Design review of the part shown in the three views and the two pictorial views. Dimensions are in mm from the part's minimum x, y and z. A direction names the side the tool comes from. Round coordinates to 2 decimals unless told otherwise and drop trailing zeros. Order: outer loops, then holes, each group sorted by start corner. A loop starts at its lowest first (then second) coordinate and runs counter-clockwise, first axis right, second up. Notation, with made-up numbers: M 76.5,68.5 L 114.5,68.5 A17 cw 114.5,84.5 Z; hole C 84,26.5 d4. An arc over 180 degrees is marked long. Write item = value, one per line. Start each with the question number.
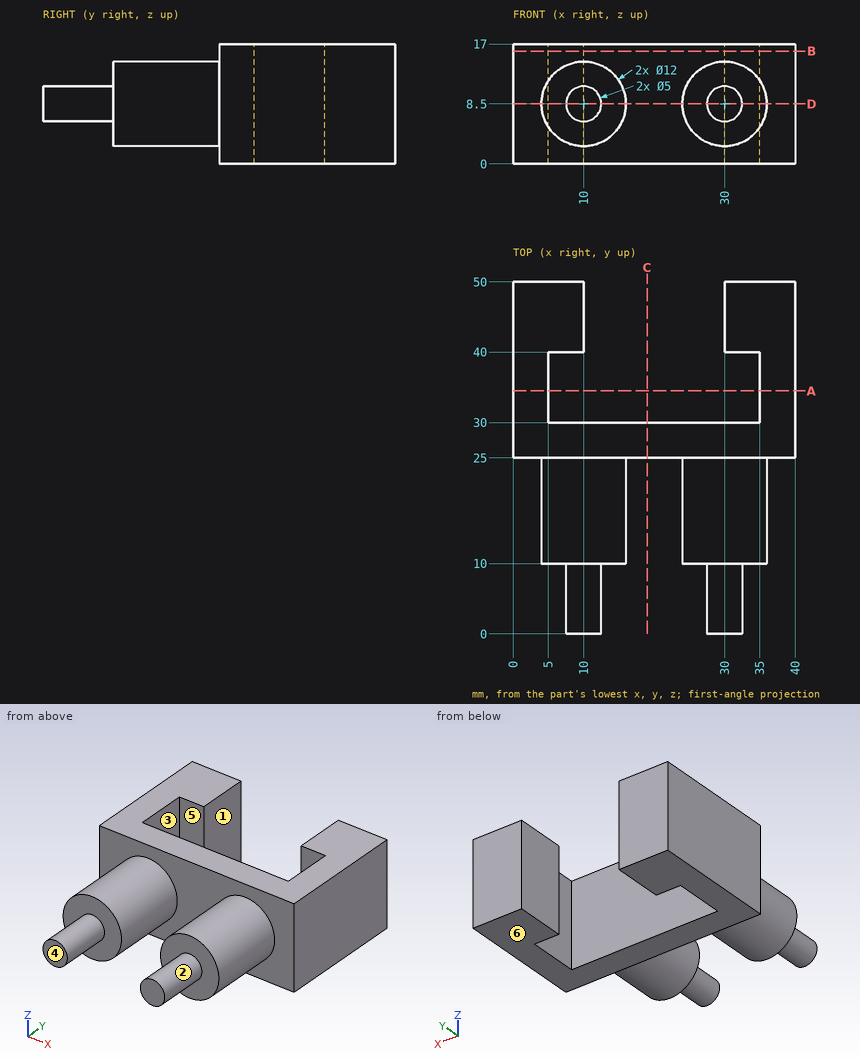
(1) For the marked faces 1, 2 and 3, list the 3-axis set-ups (+Z, -Z, +X, -X, +Y, -Y) from which the entire face can be reached by the end or side of a thin tool; tool diameter is ignored.
(2) For line 1 along X through (y, z) = (6.5, 8.75); line 2 along X through (y, z) = (31, 9.25); line 3 along Y through (x, z) = (11, 11.25), list the stretches that pass through material, from the lowest coordinate up.
(3) We need section A-A, the plane y = 34.5. Write out the cut boundary in (x, z), then the cut area to 3 significant figures.
(4) We need section B-B, the plane z = 16. Write out the cut boundary in (x, y), then the cut area to 3 significant figures.
(5) Draft analysis for pull direction Y (two halves, no side actions). For the marked faces 4, 5 and 6, state which applies: released by +Y, released by -Y, zero draft, split by the parting line, or undercut.
(6) We need section C-C, the plane x = 19. Write out the cut boundary in (y, z).
(7) We need section D-D, the plane z = 8.5. Write out the cut boundary in (x, y), then the cut area to 3 significant figures.
(8) Insertion check: pin 1 (5 mm diameter, centred on y = 47.5, z = 9.5, fed in from -X); pin 2 (2.5 mm diameter, centred on x = 7.5, z = 12.5, fed in from -Y); pin 3 (8.5 mm diameter, centred on x = 16.5, z = 5.5, fed in from +Y); pin 4 (4 mm diameter, centred on y = 22.5, z = 7.5, fed in from -X). Each pin has a flat end and moves straight along its axis. Give the tip position at first contact, or say it passes through.
Values:
q1.face_1 = +Z, -Z, +Y
q1.face_2 = -Y
q1.face_3 = +Z, -Z
q2.line_1 = 7.51 to 12.49, 27.51 to 32.49
q2.line_2 = 0 to 5, 35 to 40
q2.line_3 = 10 to 30
q3.outline = M 0,0 L 5,0 L 5,17 L 0,17 Z; M 35,0 L 40,0 L 40,17 L 35,17 Z
q3.area = 170 mm²
q4.outline = M 0,25 L 40,25 L 40,50 L 30,50 L 30,40 L 35,40 L 35,30 L 5,30 L 5,40 L 10,40 L 10,50 L 0,50 Z
q4.area = 500 mm²
q5.face_4 = released by -Y
q5.face_5 = undercut
q5.face_6 = zero draft
q6.outline = M 25,0 L 30,0 L 30,17 L 25,17 Z
q7.outline = M 0,25 L 4,25 L 4,10 L 7.5,10 L 7.5,0 L 12.5,0 L 12.5,10 L 16,10 L 16,25 L 24,25 L 24,10 L 27.5,10 L 27.5,0 L 32.5,0 L 32.5,10 L 36,10 L 36,25 L 40,25 L 40,50 L 30,50 L 30,40 L 35,40 L 35,30 L 5,30 L 5,40 L 10,40 L 10,50 L 0,50 Z
q7.area = 960 mm²
q8.pin_1 = 0
q8.pin_2 = 10
q8.pin_3 = 30
q8.pin_4 = 4
